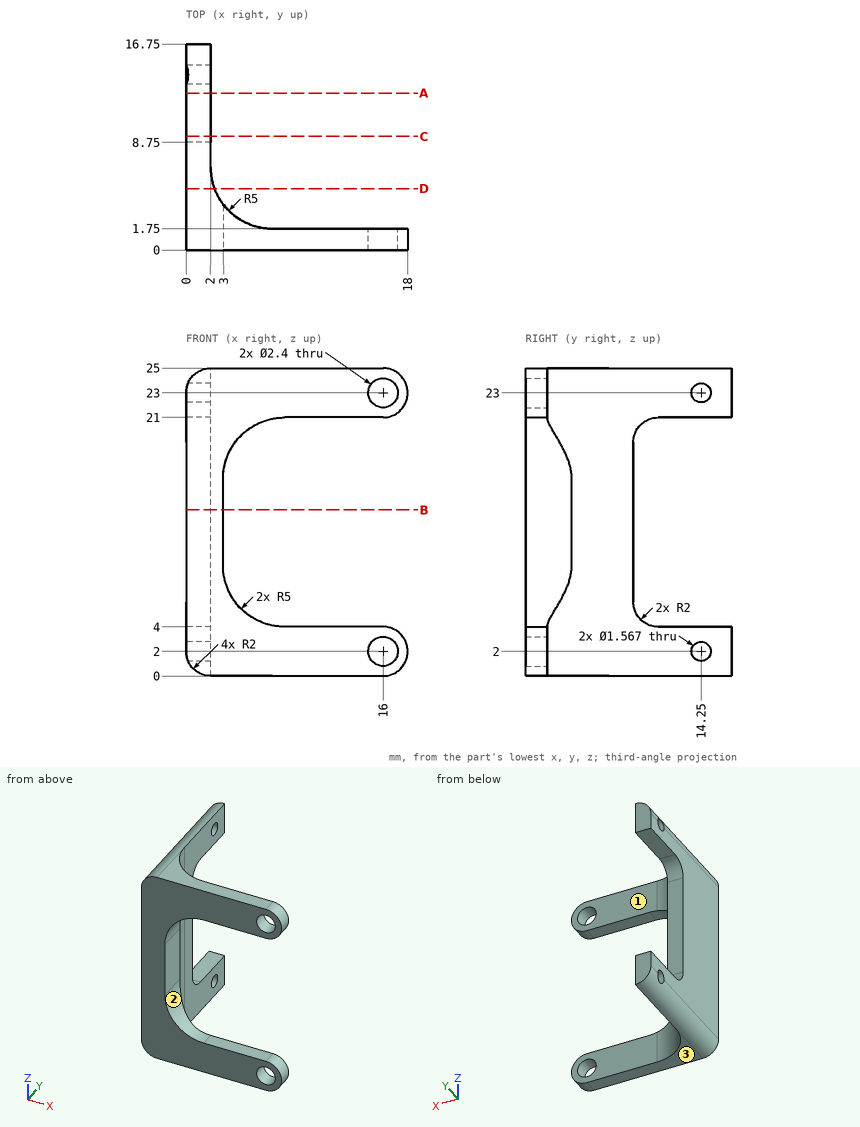
Can you work these out from the drawing? Everything is in mm from the part's minimum corner. A direction names the side the tool comes from. Round coordinates to 2 decimals unless told otherwise and drop trailing zeros. Loops run counter-clockwise (first coordinate to the right, second up) from the corner with the lowest first, then second, coordinate; pieces in that order, holes last. Notation, with made-up numbers: (-33.75, 59) -> (-26.75, 59) arc R19 cw to (-26.75, 92) -> close; hole circle Ø1 at (45, 21). An arc over 180 degrees is marked (long way). Answer in a Markdown table with one row per item.
Item 1: Suppose I cut it at D-D, the plane y = 5. List the corners of the cut face in (x, z) for me.
Answer block:
| item | result |
|---|---|
| outline | (0, 2) arc R2 ccw to (2, 0) -> (2.32, 0) -> (2.32, 25) -> (2, 25) arc R2 ccw to (0, 23) -> close |
Item 2: If I drill on probe 1 along Y at (x, z) = (1.05, 2); probe 2 along X at (y, z) = (8, 22.75); probe 3 along X at (y, z) = (0.5, 2.75), over which ranges is the centre line in solid material (lowest first)?
Answer block:
| item | result |
|---|---|
| probe 1 | 0 to 13.47, 15.03 to 16.75 |
| probe 2 | 0 to 2 |
| probe 3 | 0 to 15.06, 16.94 to 17.85 |
Item 3: Suppose I cut it at C-C, the plane y = 9.25. List the corners of the cut face in (x, z) for me, plus the area to 3 significant figures.
Answer block:
| item | result |
|---|---|
| outline | (0, 2) arc R2 ccw to (2, 0) -> (2, 4.68) -> (0, 4.68) -> close; (0, 20.32) -> (2, 20.32) -> (2, 25) arc R2 ccw to (0, 23) -> close |
| area | 17.0 mm² |
Item 4: Will these pins go through, and if not, where does the flat tip stop? P1, Ø1.8, axis at y = 14.25, z = 2, coming from the +X side; P2, Ø1.6, axis at x = 1, y = 13.5, coming from the +Z side; P3, Ø2, axis at x = 1, z = 11.5, coming from the +Y side.
Answer block:
| item | result |
|---|---|
| P1 | x = 2 |
| P2 | z = 24.99 |
| P3 | y = 8.75 |
Item 5: Suppose I cut it at B-B, the plane z = 13.5. List the corners of the cut face in (x, y) for me.
Answer block:
| item | result |
|---|---|
| outline | (0, 0) -> (3, 0) -> (3, 3.75) arc R5 cw to (2, 6.75) -> (2, 8.75) -> (0, 8.75) -> close |
Item 6: Suppose I cut it at A-A, the plane y = 12.75. List the corners of the cut face in (x, z) for me.
Answer block:
| item | result |
|---|---|
| outline | (0, 2) arc R2 ccw to (2, 0) -> (2, 4) -> (0, 4) -> close; (0, 21) -> (2, 21) -> (2, 25) arc R2 ccw to (0, 23) -> close |
Item 7: On a 3-axis mill with a long thin cutter (end or side, diameter ignored), from which of +Z, -Z, +X, -X, +Y, -Y can I reach the whole of each face in a straight line? I mean the marked faces 1, 2 and 3. Say none if no direction works.
Answer block:
| item | result |
|---|---|
| face 1 | +Z, -Z, +X, +Y |
| face 2 | +X, +Y, -Y |
| face 3 | -Z, +X, -X, +Y, -Y |
